Here's how the part is built. I have some questions about the finished solid (model axes, mm). A direction names the side the tool comes from. Round coordinates to 2 decimals unless told otherwise and drop trailing zeros. Order: outer loops, then holes, each group sorted by start corner. A loop starts at its lowest first (then second) coordinate and runs counter-clockwise, first axis right, second up. Notation, with made-up numbers: (79.5, 28.5) -> (117.5, 28.5) arc R12 cw to (117.5, 40.5) -> close; hole circle Ø7 at (0, 65.5). An arc over 180 degrees is marked (long way). Use a Markdown table: item, result. Add a question column.
from build123d import *

# Parameters (mm, degrees)
F0_R     = 9.75
F0_R_2   = 5
F0_R_3   = 1.5
F1_DEPTH = 2.5
F2_DEPTH = 0.5
F3_R     = 4.25
F3_R_2   = 1.5
F4_DEPTH = 0.5
F3_R_3   = 0.325
F5_DEPTH = 2.501


with BuildPart() as f1:
    # F0 (on Front) → F1 (new body)
    with BuildSketch(Plane.XZ):
        Circle(F0_R)
        Circle(F0_R_2, mode=Mode.SUBTRACT)
        Circle(F0_R_2)
        Circle(F0_R_3, mode=Mode.SUBTRACT)
    extrude(amount=F1_DEPTH)

    # F0 (on Front) → F2 (cut)
    with BuildSketch(Plane.XZ):
        Circle(F0_R)
        Circle(F0_R_2, mode=Mode.SUBTRACT)
    extrude(amount=F2_DEPTH, mode=Mode.SUBTRACT)

    # F3 (on face) → F4 (cut)
    with BuildSketch(Plane.XZ.offset(2.5)):
        Circle(F3_R)
        Circle(F3_R_2, mode=Mode.SUBTRACT)
    extrude(amount=-F4_DEPTH, mode=Mode.SUBTRACT)

    # F3 (on face) → F5 (cut, through all)
    with BuildSketch(Plane.XZ.offset(2.5)):
        with Locations((8.25, 0)):
            Circle(F3_R_3)
        with Locations((-8.25, 0)):
            Circle(F3_R_3)
    extrude(amount=-F5_DEPTH, mode=Mode.SUBTRACT)


solid = f1.part
(1) If we mould it in two halves opening along Z, with no side actions, what happens to faces 1 (the flat face through (4, -0.5, -4)), 2 (the cylindrical face through (2.285, -2.254, 3.584)), 3 (the cylindrical face through (-1.269, -1.486, 9.667))? For each: pulls with the +Z half, pulls with the -Z half, needs draft (parallel to the pull), parting line crosses it, or undercut.
(2) I'm going to push flat-ended pins straight in: P1, Ø7, axis at x = 0, z = 0, coming from the +Y side; P2, Ø1.5, axis at x = 1, z = 2.5, coming from the -Y side; P3, Ø2.5, axis at x = 0, z = 0, coming from the -Y side; P4, Ø1, axis at y = -1.5, z = 2.5, coming from the +X side. Where does each tip first touch, or does it pass through?
(3) I want a section at D-D on z = 2.5. List the corners of the cut face in (x, y) for me.
(4) I want a section at B-B on z = 0. List the corners of the cut face in (x, y) for me (3 decimals).
(5) On a 3-axis mill with a long thin cutter (end or side, diameter ignored), from which of +Z, -Z, +X, -X, +Y, -Y can I reach the whole of each face in a straight line? I mean faces 4 (the flat face through (-4.5, -2.5, 0.1)), 5 (the cylindrical face through (-1.08, -0.25, -4.88)), 6 (the flat face through (2, -2, 0)). Say none if no direction works.
(6) I want a section at C-C on y = -1. List the corners of the cut face in (x, z) for me (3 decimals).
(7) I want a section at A-A on x = 0. List the corners of the cut face in (y, z) for me.
(8) Please list where these lines run through material, in increasing order: probe 1 along Z at (x, y) = (0, -0.9); probe 2 along Z at (x, y) = (0, -2.2); probe 3 along Y at (x, z) = (6.5, -5.75). Write a range as from..to.
Output:
| question | item | result |
|---|---|---|
| 1 | face 1 | needs draft |
| 1 | face 2 | undercut |
| 1 | face 3 | parting line crosses it |
| 2 | P1 | y = 0 |
| 2 | P2 | y = -2 |
| 2 | P3 | through |
| 2 | P4 | x = 9.54 |
| 3 | outline | (-9.42, -2.5) -> (-3.44, -2.5) -> (-3.44, -2) -> (3.44, -2) -> (3.44, -2.5) -> (9.42, -2.5) -> (9.42, -0.5) -> (4.33, -0.5) -> (4.33, 0) -> (-4.33, 0) -> (-4.33, -0.5) -> (-9.42, -0.5) -> close |
| 4 | outline | (-9.75, -2.5) -> (-8.575, -2.5) -> (-8.575, -0.5) -> (-9.75, -0.5) -> close; (-7.925, -2.5) -> (-4.25, -2.5) -> (-4.25, -2) -> (-1.5, -2) -> (-1.5, 0) -> (-5, 0) -> (-5, -0.5) -> (-7.925, -0.5) -> close; (1.5, -2) -> (4.25, -2) -> (4.25, -2.5) -> (7.925, -2.5) -> (7.925, -0.5) -> (5, -0.5) -> (5, 0) -> (1.5, 0) -> close; (8.575, -2.5) -> (9.75, -2.5) -> (9.75, -0.5) -> (8.575, -0.5) -> close |
| 5 | face 4 | +Z, -Z, +X, -X, -Y |
| 5 | face 5 | +Y |
| 5 | face 6 | -Y |
| 6 | outline | circle Ø19.5 at (0, 0); hole circle Ø0.65 at (-8.25, 0); hole circle Ø3 at (0, 0); hole circle Ø0.65 at (8.25, 0) |
| 7 | outline | (-2.5, -9.75) -> (-0.5, -9.75) -> (-0.5, -5) -> (0, -5) -> (0, -1.5) -> (-2, -1.5) -> (-2, -4.25) -> (-2.5, -4.25) -> close; (-2.5, 4.25) -> (-2, 4.25) -> (-2, 1.5) -> (0, 1.5) -> (0, 5) -> (-0.5, 5) -> (-0.5, 9.75) -> (-2.5, 9.75) -> close |
| 8 | probe 1 | -9.75..-1.5, 1.5..9.75 |
| 8 | probe 2 | -9.75..-4.25, 4.25..9.75 |
| 8 | probe 3 | -2.5..-0.5 |
